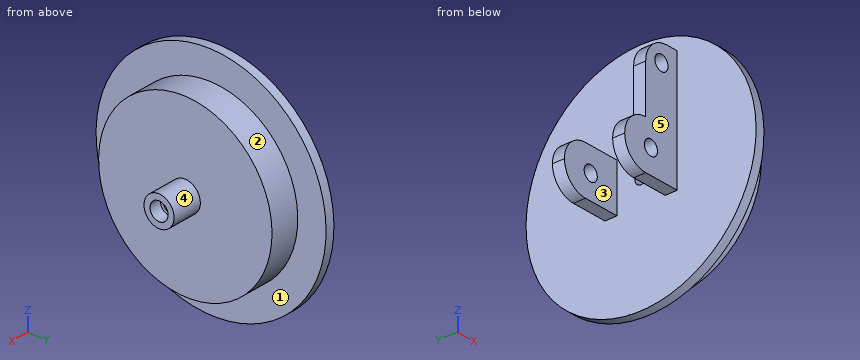
from build123d import *

# Parameters (mm, degrees)
SKETCH2_R           = 1
CUT_EXTRUDE1_DEPTH  = 30.321700517
SKETCH3_R           = 1.5
CUT_EXTRUDE2_DEPTH  = 2
SKETCH4_W           = 8
SKETCH4_H           = 2
BOSS_EXTRUDE1_DEPTH = 10
SKETCH6_R           = 1.25
CUT_EXTRUDE4_DEPTH  = 20
FILLET1_R           = 4
SKETCH7_W           = 6
SKETCH7_H           = 2
BOSS_EXTRUDE2_DEPTH = 12
SKETCH8_R           = 1.25
CUT_EXTRUDE5_DEPTH  = 12
FILLET2_R           = 4


with BuildPart() as part:
    # Sketch1 → Revolve1 (revolve)
    with BuildSketch(Plane(origin=(0, 0, 0), x_dir=(1, 0, 0), z_dir=(0, 1, 0)), mode=Mode.PRIVATE) as revolve1_sk:
        Polygon((0, 2.5), (0, 14.4), (-4.907984975, 14.4), (-4.907984975, 19.1), (-6.407984975, 19.1), (-6.407984975, 0), (0, 0), (5, 0), (5, 2.5), align=None)
    revolve(revolve1_sk.sketch.rotate(Axis((-25.527114743, 0, 0), (1, 0, 0)), 180), axis=Axis((-25.527114743, 0, 0), (1, 0, 0)))

    # Sketch2 → Cut-Extrude1 (cut, through all)
    with BuildSketch(Plane.ZY.offset(6.407984975)):
        Circle(SKETCH2_R)
    extrude(amount=-CUT_EXTRUDE1_DEPTH, mode=Mode.SUBTRACT)

    # Sketch3 → Cut-Extrude2 (cut)
    with BuildSketch(Plane(origin=(5, 0, 0), x_dir=(0, 0, -1), z_dir=(1, 0, 0))):
        Circle(SKETCH3_R)
    extrude(amount=-CUT_EXTRUDE2_DEPTH, mode=Mode.SUBTRACT)

    # Sketch4 → Boss-Extrude1 (add)
    with BuildSketch(Plane.ZY.offset(6.407984975)):
        with Locations((0, 5)):
            Rectangle(SKETCH4_W, SKETCH4_H)
        with Locations((0, -5)):
            Rectangle(SKETCH4_W, SKETCH4_H)
    extrude(amount=BOSS_EXTRUDE1_DEPTH)

    # Sketch6 → Cut-Extrude4 (cut)
    with BuildSketch(Plane(origin=(0, 6, 0), x_dir=(1, 0, 0), z_dir=(0, 1, 0))):
        with Locations(Location((-11.407984975, 0, 0), (0, 0, 270))):
            Circle(SKETCH6_R)
    extrude(amount=-CUT_EXTRUDE4_DEPTH, mode=Mode.SUBTRACT)

    # Fillet1
    fillet1_edges = [part.edges().sort_by_distance(p)[0] for p in [
        (-16.407984975, -5, 4),
        (-16.407984975, -5, -4),
        (-16.407984975, 5, 4),
        (-16.407984975, 5, -4),
    ]]
    fillet(fillet1_edges, radius=FILLET1_R - 0.0001)  # a hair under: the kernel refuses the full size

    # Sketch7 → Boss-Extrude2 (add)
    with BuildSketch(Plane.XY.offset(4)):
        with Locations((-9.407984975, -5)):
            Rectangle(SKETCH7_W, SKETCH7_H)
    extrude(amount=BOSS_EXTRUDE2_DEPTH)

    # Sketch8 → Cut-Extrude5 (cut)
    with BuildSketch(Plane(origin=(0, -4, 0), x_dir=(1, 0, 0), z_dir=(0, 1, 0))):
        with Locations(Location((-9.407984975, -13, 0), (0, 0, 270))):
            Circle(SKETCH8_R)
    extrude(amount=-CUT_EXTRUDE5_DEPTH, mode=Mode.SUBTRACT)

    # Fillet2
    fillet2_edges = [part.edges().sort_by_distance(p)[0] for p in [
        (-12.407984975, -5, 16),
    ]]
    fillet(fillet2_edges, radius=FILLET2_R)


solid = part.part
Geometry check sheet. Reference: the model listing, model coordinates, mm. Face numbers are marked on the shaded views. A direction names the side the tool comes from. Give positions to 0.01 mm unless a question says otherwise; leave off trailing zeros. Write each loop counter-clockwise with the first axis right and the second up, starting at its lowest first coordinate (ties: lowest second). Pieces come first, ordered by that corner, then holes. Notation, with made-up numbers: (-17, 16) - (22, 16) arc R18 cw to (22, 32) - close; hole circle Ø9 at (66.5, 72.25). An arc over 180 degrees is marked (long way). Put each result on its own line as item: value.
1. Thickness scan on line 1 (X direction, y = -5, z = 0); line 2 (Y direction, x = -7.75, z = 1.5); line 3 (Y direction, x = 4.6, z = 0). Record the ranges inside material, lowest first.
Ans:
line 1: x = -16.41 to -12.66, -10.16 to 0
line 2: y = -6 to -4, 4 to 6
line 3: y = -2.5 to -1.5, 1.5 to 2.5
2. Sectioned sample at C-C, the plane y = 8. Enter the section's corners in (x, z).
Ans:
outline: (-6.41, -17.34) - (-4.91, -17.34) - (-4.91, -11.97) - (0, -11.97) - (0, 11.97) - (-4.91, 11.97) - (-4.91, 17.34) - (-6.41, 17.34) - close
3. Set-up check for the marked faces 4 and 5: record each of +Z, -Z, +X, -X, +Y, -Y from which the full face is reachable in a straight line by a thin tool's end or side.
Ans:
face 4: +X
face 5: +Z, -Z, -X, -Y
4. Sectioned sample at B-B, the plane x = -1.5. Enter the section's corners in (y, z).
Ans:
outline: circle Ø28.8 at (0, 0); hole circle Ø2 at (0, 0)
5. Sectioned sample at A-A, the plane z = 13. Enter the section's corners in (x, y), plus the area to 3 significant figures.
Ans:
outline: (-12.28, -6) - (-10.66, -6) - (-10.66, -4) - (-12.28, -4) - close; (-8.16, -6) - (-6.41, -6) - (-6.41, -13.99) - (-4.91, -13.99) - (-4.91, -6.19) - (0, -6.19) - (0, 6.19) - (-4.91, 6.19) - (-4.91, 13.99) - (-6.41, 13.99) - (-6.41, -4) - (-8.16, -4) - close
area: 110 mm²
6. Sectioned sample at D-D, the plane z = 6. Enter the section's corners in (x, y).
Ans:
outline: (-12.41, -6) - (-6.41, -6) - (-6.41, -18.13) - (-4.91, -18.13) - (-4.91, -13.09) - (0, -13.09) - (0, 13.09) - (-4.91, 13.09) - (-4.91, 18.13) - (-6.41, 18.13) - (-6.41, -4) - (-12.41, -4) - close
7. Go/stop test with flat-tipped pins: pin 1 (5 mm diameter, centred on x = -7.5, z = -7.5, fed in from +Y); pin 2 (9 mm diameter, centred on x = -13, z = 1, fed in from -Y); pin 3 (1 mm diameter, centred on y = 3, z = 14.5, fed in from +X). Record where each tip stops, or that it passes through.
Ans:
pin 1: stops at y = 18.36
pin 2: stops at y = -6
pin 3: stops at x = 0
8. Draft check along Y on the marked faces 1, 2 and 3. Enter one of: +Y half, -Y half, draft (parallel to the pull), parting line (faces both ways), or undercut.
Ans:
face 1: draft
face 2: parting line
face 3: undercut
